```python
from build123d import *

# Parameters (mm, degrees)
SKETCH1_R      = 4.9911
EXTRUDE1_DEPTH = 1.0922
SKETCH2_R      = 1.27
EXTRUDE2_DEPTH = 10.16
SKETCH3_R      = 2.54
EXTRUDE3_DEPTH = 7.62
SKETCH4_R      = 1.7272
EXTRUDE4_DEPTH = 3.175
FILLET1_R      = 1.524
CHAMFER4_SIZE  = 0.762
FILLET2_R      = 1.016


with BuildPart() as part:
    # Sketch1 → Extrude1 (new body)
    with BuildSketch(Plane.XY):
        Circle(SKETCH1_R)
    extrude(amount=EXTRUDE1_DEPTH)

    # Sketch2 → Extrude2 (add)
    with BuildSketch(Plane.XY.offset(1.0922)):
        Circle(SKETCH2_R)
    extrude(amount=EXTRUDE2_DEPTH)

    # Sketch3 → Extrude3 (add)
    with BuildSketch(Plane.XY.offset(11.2522)):
        Circle(SKETCH3_R)
    extrude(amount=-EXTRUDE3_DEPTH)

    # Sketch4 → Extrude4 (add)
    with BuildSketch(Plane.XY.offset(11.2522)):
        Circle(SKETCH4_R)
    extrude(amount=EXTRUDE4_DEPTH)

    # Fillet1
    fillet1_edges = [part.edges().sort_by_distance(p)[0] for p in [
        (-1.7272, 0, 14.4272),
    ]]
    fillet(fillet1_edges, radius=FILLET1_R)

    # Chamfer4
    chamfer4_edges = [part.edges().sort_by_distance(p)[0] for p in [
        (-2.54, 0, 11.2522),
    ]]
    chamfer(chamfer4_edges, length=CHAMFER4_SIZE)

    # Fillet2
    fillet2_edges = [part.edges().sort_by_distance(p)[0] for p in [
        (-4.9911, 0, 0),
    ]]
    fillet(fillet2_edges, radius=FILLET2_R)


solid = part.part
```
Part model, mm, in its own coordinate system. A direction names the side the tool comes from. Round coordinates to 2 decimals unless told otherwise and drop trailing zeros. Order: outer loops, then holes, each group sorted by start corner. A loop starts at its lowest first (then second) coordinate and runs counter-clockwise, first axis right, second up. Notation, with made-up numbers: M 36,7.25 L 71,7.25 A19 cw 71,36.25 Z; hole C 18,54.5 d11. An arc over 180 degrees is marked long. Answer in a Markdown table with one row per item. Add a question column.
Q1. Wall check: L1, parallel to Z at x = -3.25, y = 1; L2, parallel to Z at x = 1.75, y = 1.5; L3, parallel to Z at x = 4.25, y = 1.5. Give the ranges that are in metal, low to high. Write a range as from..to.
Q2. Mould opens along Z. For faces 3 (the face through (0, 0, 0)), 4 (the face through (-0.33, 2.52, 7.11)), 5 (the face through (-0.17, 1.26, 2.34)) say: +Z half, -Z half, draft (parallel to the pull), parting line (faces both ways), or undercut.
Q3. Pin check, flat tips, straight feed: pin 1 (4 mm diameter, centred on y = -2.5, z = 7.5, fed in from +X); pin 2 (3 mm diameter, centred on x = -2.5, z = 4.5, fed in from +Y); pin 3 (5 mm diameter, centred on y = 2.5, z = 2.5, fed in from +X); pin 4 (4 mm diameter, centred on x = 0.5, y = 0.5, fed in from +Z). Stop position of each tip, or through.
Q4. Cut at A-A on z = 8.5. Give the cut face in (x, y), and give its area (3 significant figures).
Q5. 3-axis set-ups, long thin cutter, end or side, ignore diameter. For faces 1 (the face through (-0.225, 1.713, 12.066)), 2 (the face through (1.04, -1.04, 1.092)): which of +Z, -Z, +X, -X, +Y, -Y reach the whole face in a straight line?
Q6. Cut at B-B on z = 10.75. Give the cut face in (x, y).
Established:
| question | item | result |
|---|---|---|
| 1 | L1 | z = 0..1.09 |
| 1 | L2 | z = 0..1.09, 3.63..10.73 |
| 1 | L3 | z = 0.15..1.09 |
| 2 | face 3 | -Z half |
| 2 | face 4 | draft |
| 2 | face 5 | undercut |
| 3 | pin 1 | stops at x = 2.49 |
| 3 | pin 2 | stops at y = 2.33 |
| 3 | pin 3 | stops at x = 4.97 |
| 3 | pin 4 | stops at z = 14.43 |
| 4 | outline | C 0,0 d5.08 |
| 4 | area | 20.3 mm2 |
| 5 | face 1 | +Z |
| 5 | face 2 | none |
| 6 | outline | C 0,0 d4.56 |
